from build123d import *

# Parameters (mm, degrees)
CROQUIS1_W              = 1000
CROQUIS1_H              = 30
SALIENTE_EXTRUIR1_DEPTH = 20
CORTAR_EXTRUIR1_DEPTH   = 1001.649788887
CROQUIS3_W              = 100
CROQUIS3_H              = 30
CORTAR_EXTRUIR2_DEPTH   = 502.29831438
CROQUIS4_R              = 5
CORTAR_EXTRUIR3_DEPTH   = 10


with BuildPart() as part:
    # Croquis1 → Saliente-Extruir1 (new body)
    with BuildSketch(Plane.XY):
        with Locations((0, 15)):
            Rectangle(CROQUIS1_W, CROQUIS1_H)
    extrude(amount=SALIENTE_EXTRUIR1_DEPTH)

    # Croquis2 → Cortar-Extruir1 (cut, through all)
    with BuildSketch(Plane(origin=(500, 0, 0), x_dir=(0, 0, -1), z_dir=(1, 0, 0))):
        Polygon((-17, 27), (-17, 3), (-3, 3), (-3, 12.998729457), (0, 12.998729457), (0, 17), (-3, 17), (-3, 27), align=None)
    extrude(amount=-CORTAR_EXTRUIR1_DEPTH, mode=Mode.SUBTRACT)

    # Croquis3 → Cortar-Extruir2 (cut, through all)
    with BuildSketch(Plane.XY.offset(20)):
        with Locations((-450, 15)):
            Rectangle(CROQUIS3_W, CROQUIS3_H)
        with Locations((450, 15)):
            Rectangle(CROQUIS3_W, CROQUIS3_H)
    extrude(amount=-CORTAR_EXTRUIR2_DEPTH, mode=Mode.SUBTRACT)

    # Croquis4 → Cortar-Extruir3 (cut)
    with BuildSketch(Plane.XY.offset(20)):
        with Locations((300, 15)):
            Circle(CROQUIS4_R)
        with Locations((0, 15)):
            Circle(CROQUIS4_R)
        with Locations((-283.92, 15)):
            Circle(CROQUIS4_R)
    extrude(amount=-CORTAR_EXTRUIR3_DEPTH, mode=Mode.SUBTRACT)


solid = part.part
Geometry: final body of the model. Coordinates: model frame, mm. A direction names the side the tool comes from. Coordinates: 2 decimals unless noted, no trailing zeros. Loops run counter-clockwise (first coordinate to the right, second up) from the corner with the lowest first, then second, coordinate; pieces in that order, holes last. Notation, with made-up numbers: M 38.5,51.25 L 67.5,51.25 A11 cw 67.5,60.25 Z; hole C 73.5,37.5 d5. An arc over 180 degrees is marked long. One line per item, written item: value. Start each with the question number.
1) Material intervals for L1, parallel to Y at x = -108.5, z = 8.5; L2, parallel to Y at x = 0, z = 18.7; L3, parallel to Z at x = -60, y = 6, sorted ascending. Write a range as from..to.
2) Cut plane B-B (x = -79.5). Return loops of the section in (y, z), then the cut area to 3 significant figures.
3) Pin query (flat end, axial travel): P1, Ø9, axis at x = 0, y = 15, coming from the +Z side; P2, Ø4, axis at x = -41.5, z = 11, coming from the -Y side. Return the tip coordinate at first contact, or that it passes through.
4) Reachability of faces 4 (the flat face through (6, 15, 17)), 5 (the flat face through (-400, 15, 19)) from +Z, -Z, +X, -X, +Y, -Y: full face, straight path, thin tool, end or side. Return the list, or none.
5) Cut plane A-A (z = 11.75). Return loops of the section in (x, y), then the cut area to 3 significant figures.
6) Draft query along Y for faces 1 (the flat face through (6, 3, 10)), 2 (the flat face through (400, 15, 19)), 3 (the flat face through (-6, 0, 10)). Return one class per face: released by +Y, released by -Y, zero draft, split by the parting line, or undercut.
Evaluation:
1. L1: 0..3, 27..30
1. L2: 0..10, 20..30
1. L3: 0..3, 17..20
2. outline: M 0,0 L 13,0 L 13,3 L 3,3 L 3,17 L 27,17 L 27,3 L 17,3 L 17,0 L 30,0 L 30,20 L 0,20 Z
2. area: 252 mm^2
3. P1: z = 3
3. P2: y = 0
4. face 4: +X, -X
4. face 5: +Z, -Z, -X, +Y, -Y
5. outline: M -400,0 L 400,0 L 400,3 L -400,3 Z; M -400,27 L 400,27 L 400,30 L -400,30 Z
5. area: 4,800 mm^2
6. face 1: undercut
6. face 2: zero draft
6. face 3: released by -Y
